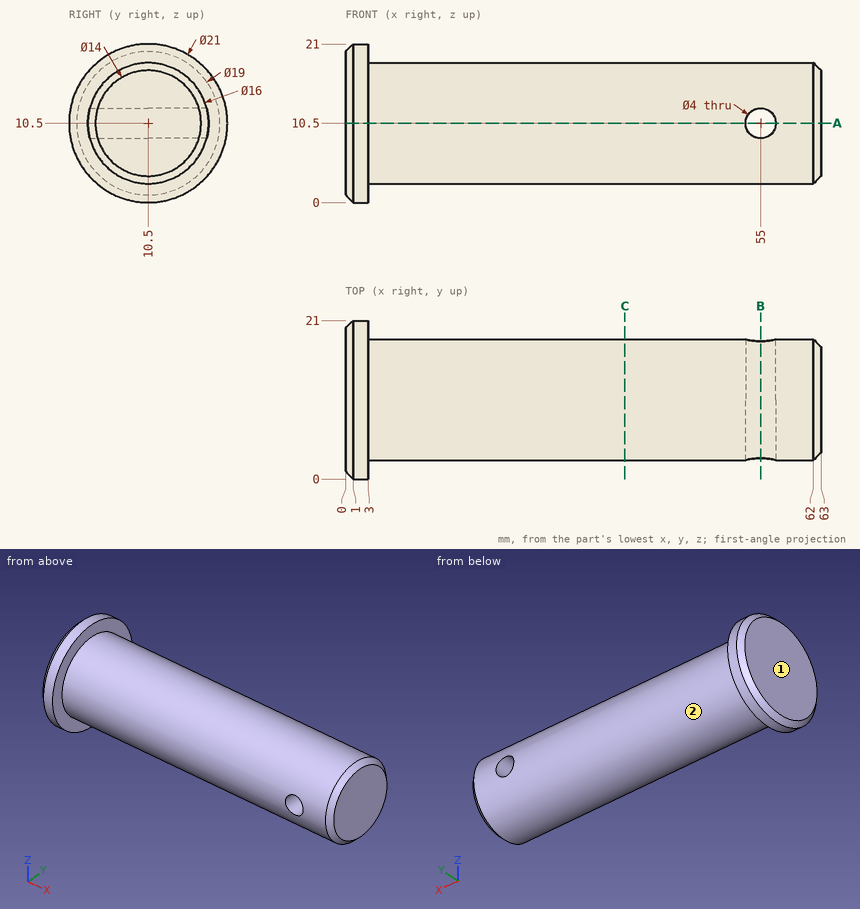
Drawing for the job (mm, zero at the part's lowest x, y, z). A direction names the side the tool comes from. Coordinates: 2 decimals unless noted, no trailing zeros. Order: outer loops, then holes, each group sorted by start corner. A loop starts at its lowest first (then second) coordinate and runs counter-clockwise, first axis right, second up. Notation, with made-up numbers: (48, 86.5) -> (99, 86.5) arc R16 cw to (99, 108.5) -> close; hole circle Ø2 at (36.5, 64). An arc over 180 degrees is marked (long way). One line per item, written item: value.
(1) Slice it at A-A, the plane z = 10.5. List the corners of the cut face in (x, y).
Checked values:
outline: (0, 1) -> (1, 0) -> (3, 0) -> (3, 2.5) -> (53, 2.5) -> (53, 18.5) -> (3, 18.5) -> (3, 21) -> (1, 21) -> (0, 20) -> close; (57, 2.5) -> (62, 2.5) -> (63, 3.5) -> (63, 17.5) -> (62, 18.5) -> (57, 18.5) -> close
(2) Slice it at B-B, the plane x = 55. List the corners of the cut face in (y, z).
Checked values:
outline: (2.75, 8.5) arc R8 ccw to (18.25, 8.5) -> close; (2.75, 12.5) -> (18.25, 12.5) arc R8 ccw to start
(3) Slice it at C-C, the plane x = 37. List the corners of the cut face in (y, z), plus the area to 3 significant figures.
Checked values:
outline: circle Ø16 at (10.5, 10.5)
area: 201 mm2
(4) Probe line 1 (X direction, y = 8, z = 10.5); line 2 (X direction, y = 10.75, z = 17.5); line 3 (Z direction, x = 55, y = 14.25). List the from-to ranges inside material, lowest first. Write a range as [from, to].
Checked values:
line 1: [0, 53], [57, 63]
line 2: [0, 63]
line 3: [3.43, 8.5], [12.5, 17.57]
(5) Tool access for the marked faces 1 and 2: list every direction of +Z, -Z, +X, -X, +Y, -Y with a clear straight run to the whole face (end or side of a thin tool).
Checked values:
face 1: +Z, -Z, -X, +Y, -Y
face 2: +X
(6) Drop flat-ended pins along their axis: pin 1 Ø6.5 at (x, z) = (55, 10.5) entering from +Y; pin 2 Ø8 at (x, z) = (25.5, 15.5) entering from +Y; pin 3 Ø12 at (x, y) = (56.5, 3.5) entering from +Z. Give the stop position or say it passes through.
Checked values:
pin 1: y = 18.5
pin 2: y = 18.44
pin 3: z = 18.44
